from build123d import *

# Parameters (mm, degrees)
SKETCH1_W                                            = 119.888
SKETCH1_H                                            = 86.36
BOSS_EXTRUDE1_DEPTH                                  = 4.572
CBORE_FOR_M3_HEXAGON_SOCKET_HEAD_CAP_SCR_D           = 3.4
CBORE_FOR_M3_HEXAGON_SOCKET_HEAD_CAP_SCR_CBORE_D     = 6
CBORE_FOR_M3_HEXAGON_SOCKET_HEAD_CAP_SCR_CBORE_DEPTH = 3.4
SKETCH5_R                                            = 3.175
CUT_EXTRUDE1_DEPTH                                   = 5.572


with BuildPart() as part:
    # Sketch1 → Boss-Extrude1 (new body)
    with BuildSketch(Plane(origin=(0, 0, 0), x_dir=(1, 0, 0), z_dir=(0, 1, 0))):
        Rectangle(SKETCH1_W, SKETCH1_H)
    extrude(amount=BOSS_EXTRUDE1_DEPTH)

    # CBORE for M3 Hexagon socket head cap screws1 (through all)
    with Locations(Plane(origin=(0, 4.572, 0), x_dir=(1, 0, 0), z_dir=(0, 1, 0))):
        with Locations((8.128, 38.1), (12.827, -39.37), (-12.827, -39.37), (-8.128, 38.1)):
            CounterBoreHole(CBORE_FOR_M3_HEXAGON_SOCKET_HEAD_CAP_SCR_D / 2, CBORE_FOR_M3_HEXAGON_SOCKET_HEAD_CAP_SCR_CBORE_D / 2, CBORE_FOR_M3_HEXAGON_SOCKET_HEAD_CAP_SCR_CBORE_DEPTH)

    # Sketch5 → Cut-Extrude1 (cut, through all)
    with BuildSketch(Plane(origin=(0, 4.572, 0), x_dir=(1, 0, 0), z_dir=(0, 1, 0))):
        with Locations((50.8, 25.225713352)):
            Circle(SKETCH5_R)
        with Locations((50.8, -25.574286648)):
            Circle(SKETCH5_R)
        with Locations((-50.8, 25.225713352)):
            Circle(SKETCH5_R)
        with Locations((-50.8, -25.574286648)):
            Circle(SKETCH5_R)
    extrude(amount=-CUT_EXTRUDE1_DEPTH, mode=Mode.SUBTRACT)


solid = part.part
Design review of the part built by this model. Coordinates are the model's own, in mm. A direction names the side the tool comes from. Coordinates: 2 decimals unless noted, no trailing zeros. Order: outer loops, then holes, each group sorted by start corner. A loop starts at its lowest first (then second) coordinate and runs counter-clockwise, first axis right, second up. Notation, with made-up numbers: (38, 11.25) -> (72, 11.25) arc R6 ccw to (72, 15.25) -> close; hole circle Ø6 at (33, 7.5). An arc over 180 degrees is marked (long way). One line per item, written item: value.
1) Draft analysis for pull direction X (two halves, no side actions). For faces 3 (the face through (59.944, 2, 1)), 4 (the face through (-1, 0, -1)), 5 (the face through (-13.48, 2.9, 42.3)), state which applies: +X half, -X half, draft (parallel to the pull), parting line (faces both ways), or undercut.
Output values:
face 3: +X half
face 4: draft
face 5: undercut
2) We need section C-C, the plane y = 3.1. Count the separate pieces of the cut face and the enclosed holes in it, then the cut area to 3 significant figures.
Output values:
separate pieces: 1
enclosed holes: 8
area: 10,100 mm2
3) We need section B-B, the plane z = 39.37. Give the boundary of the cut face in (x, y).
Output values:
outline: (-59.94, 0) -> (-14.53, 0) -> (-14.53, 1.17) -> (-15.83, 1.17) -> (-15.83, 4.57) -> (-59.94, 4.57) -> close; (-11.13, 0) -> (11.13, 0) -> (11.13, 1.17) -> (9.83, 1.17) -> (9.83, 4.57) -> (-9.83, 4.57) -> (-9.83, 1.17) -> (-11.13, 1.17) -> close; (14.53, 0) -> (59.94, 0) -> (59.94, 4.57) -> (15.83, 4.57) -> (15.83, 1.17) -> (14.53, 1.17) -> close
4) Machinability: for faces 1 (the face through (53.733, 2.318, -24.01)), 2 (the face through (-6.8, 1.172, -36.8)), which of the approach directions +Z, -Z, +X, -X, +Y, -Y give a long, thin tool a straight path to every point of the face, cutting with its end or side? Answer none if there is none.
Output values:
face 1: +Y, -Y
face 2: +Y
5) To check wall thickness, follow probe 1 along X at (y, z) = (0.8, -38.1); probe 2 along Z at (x, y) = (-13, 3.3) (3 decimals); probe 3 along Z at (x, y) = (-50.8, 1.15). State the ranges of each line that lie inside material, in increasing order. Write a range as [from, to].
Output values:
probe 1: x = [-59.94, -9.83], [-6.43, 6.43], [9.83, 59.94]
probe 2: z = [-43.18, 36.375], [42.365, 43.18]
probe 3: z = [-43.18, -28.4], [-22.05, 22.4], [28.75, 43.18]
6) Clearance check with a flat-ended pin moving along its axis: P1, Ø5, axis at x = -8.128, z = -38.1, coming from the +Y side. State where the tip first meets the part, or that it passes through.
Output values:
P1: stops at y = 1.17
7) We need section A-A, the plane x = 50.8. Give the boundary of the cut face in (y, z).
Output values:
outline: (0, -43.18) -> (4.57, -43.18) -> (4.57, -28.4) -> (0, -28.4) -> close; (0, -22.05) -> (4.57, -22.05) -> (4.57, 22.4) -> (0, 22.4) -> close; (0, 28.75) -> (4.57, 28.75) -> (4.57, 43.18) -> (0, 43.18) -> close
